The figure shows three views and two pictorial views of one solid part (mm, origin at its lowest corner). Answer the questions. A direction names the side the tool comes from. Give positions to 0.01 mm unless a question says otherwise; leave off trailing zeros. Loops run counter-clockwise (first coordinate to the right, second up) from the corner with the lowest first, then second, coordinate; pieces in that order, holes last. Notation, with made-up numbers: (65, 76) - (117, 76) arc R20 ccw to (117, 109) - close; hole circle Ø6 at (-3.5, -25.5). An arc over 180 degrees is marked (long way). Use CSV: the item, a comma, the result in double quotes.
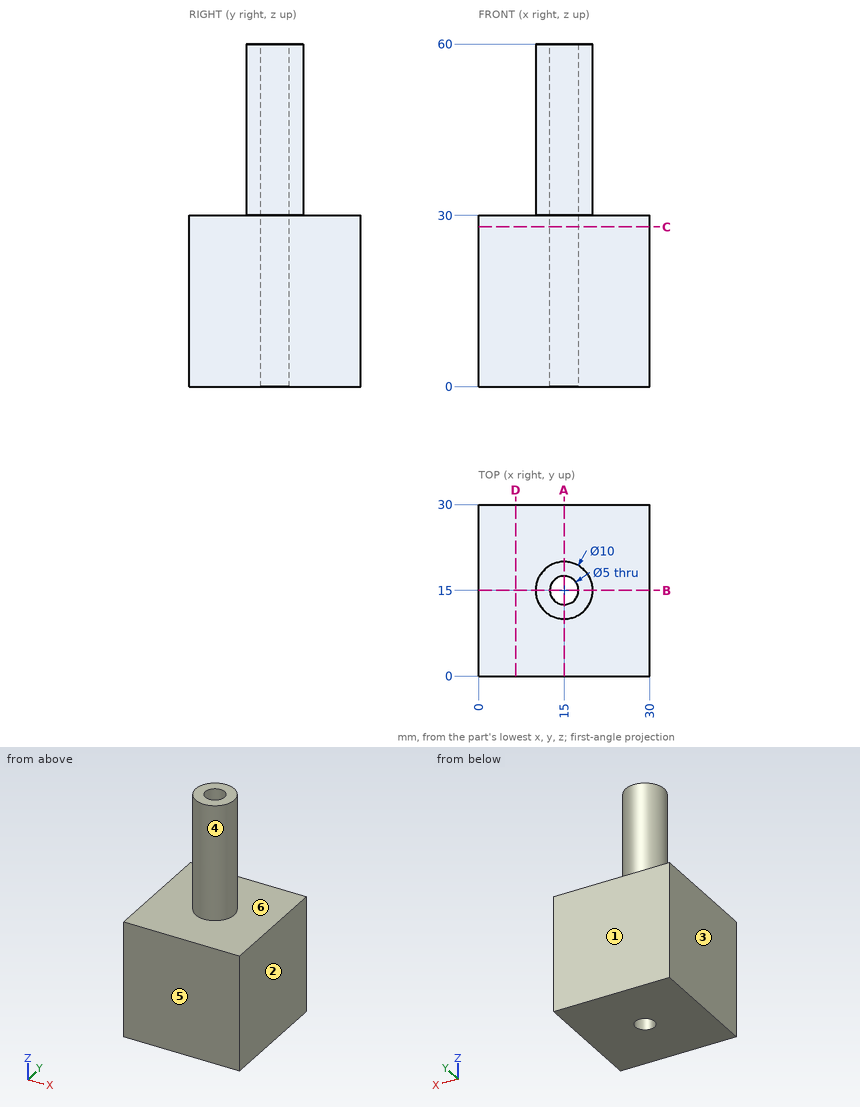
Item 1: The mould has two halves that part along X. Classify the marked faces 1, 2, 3 and 4: pulls with the +X half, pulls with the -X half, needs draft (parallel to the pull), parting line crosses it, or undercut.
Determined:
face 1,"needs draft"
face 2,"pulls with the +X half"
face 3,"pulls with the -X half"
face 4,"parting line crosses it"
Item 2: A cutting plane is placed at A-A on x = 15. Determine the outline of the cut face in (y, z).
Determined:
outline,"(0, 0) - (12.5, 0) - (12.5, 60) - (10, 60) - (10, 30) - (0, 30) - close; (17.5, 0) - (30, 0) - (30, 30) - (20, 30) - (20, 60) - (17.5, 60) - close"
Item 3: For the marked faces 5 and 6, determine the directions among +Z, -Z, +X, -X, +Y, -Y from which every point of the face is accessible in a straight line to the end or side of a thin tool.
Determined:
face 5,"+Z, -Z, +X, -X, -Y"
face 6,"+Z"
Item 4: Find the intervals of material crossed by line 1 (Y direction, x = 15, z = 35.5); line 2 (Z direction, x = 12, y = 22); line 3 (Y direction, x = 17.25, z = 13), in increasing order.
Determined:
line 1,"y = 10 to 12.5, 17.5 to 20"
line 2,"z = 0 to 30"
line 3,"y = 0 to 13.91, 16.09 to 30"
Item 5: A cutting plane is placed at D-D on x = 6.5. Determine the outline of the cut face in (y, z), and give its area (3 significant figures).
Determined:
outline,"(0, 0) - (30, 0) - (30, 30) - (0, 30) - close"
area,"900 mm²"
Item 6: A cutting plane is placed at C-C on z = 28. Determine the outline of the cut face in (x, y), and give its area (3 significant figures).
Determined:
outline,"(0, 0) - (30, 0) - (30, 30) - (0, 30) - close; hole circle Ø5 at (15, 15)"
area,"880 mm²"
Item 7: Given P1, Ø10, axis at y = 3.5, z = 9.5, coming from the -X side; P2, Ø4, axis at x = 18, y = 5.5, coming from the +Z side, each flat-ended and moving along its own axis, determine where each tip first touches the part or whether it passes through.
Determined:
P1,"stops at x = 0"
P2,"stops at z = 30"
